Autodesk Fusion 360 part; units mm, degrees
ref_plane "WorkPlane3" through (0, 0, -38) normal (0, 0, 1) x (1, 0, 0)
sketch "Sketch6" plane through (0, 0, -38) normal (0, 0, 1) x (1, 0, 0)
  line L0 (-34.25, -21.25) -> (34.25, -21.25)
  line L1 (34.25, -21.25) -> (34.25, 21.25)
  line L2 (34.25, 21.25) -> (-34.25, 21.25)
  line L3 (-34.25, 21.25) -> (-34.25, -21.25)
extrude "Extrude6" add sketch "Sketch6" along normal blind 30
fillet "Fillet7" radius 2.5 4 edges at (-34.25, 21.25, -23) (34.25, 21.25, -23) (34.25, -21.25, -23) (-34.25, -21.25, -23)
ref_plane "WorkPlane4" through (0, 0, -8) normal (0, 0, 1) x (1, 0, 0)
sketch "Sketch7" plane through (0, 0, -8) normal (0, 0, 1) x (1, 0, 0)
  line L0 (-44.25, -31.25) -> (44.25, -31.25)
  line L1 (44.25, -31.25) -> (44.25, 90)
  line L2 (44.25, 90) -> (-44.25, 90)
  line L3 (-44.25, 90) -> (-44.25, -31.25)
extrude "Extrude7" add sketch "Sketch7" along normal blind 12
fillet "Fillet8" radius 7 4 edges at (-44.25, 90, -2) (44.25, 90, -2) (44.25, -31.25, -2) (-44.25, -31.25, -2)
sketch "Sketch8" plane through (0, 0, -8) normal (0, 0, 1) x (1, 0, 0)
  line L0 (-34.547, 90) -> (-11.5, 50.0814)
  arc A0 (-11.5, 50.0814) -> (11.5, 50.0814) centre (0, 70) ccw
  line L1 (11.5, 50.0814) -> (34.547, 90)
  line L2 (34.547, 90) -> (34.547, 95)
  line L3 (34.547, 95) -> (-34.547, 95)
  line L4 (-34.547, 95) -> (-34.547, 90)
extrude "Extrude8" cut sketch "Sketch8" along normal blind 12
fillet "Fillet9" radius 5 64 edges at (33.5178, -20.5178, -8) (0, -21.25, -8) (-33.5178, -20.5178, -8) (-34.25, 0, -8) (-33.5178, 20.5178, -8) (0, 21.25, -8) (33.5178, 20.5178, -8) (34.25, 0, -8) (34.25, 0, -8) (33.5178, 20.5178, -8) (0, 21.25, -8) (-33.5178, 20.5178, -8) (-34.25, 0, -8) (-33.5178, -20.5178, -8) (0, -21.25, -8) (33.5178, -20.5178, -8) (33.5178, 20.5178, -8) (34.25, 0, -8) (33.5178, -20.5178, -8) (0, -21.25, -8) (-33.5178, -20.5178, -8) (-34.25, 0, -8) (-33.5178, 20.5178, -8) (0, 21.25, -8) (0, 21.25, -8) (-33.5178, 20.5178, -8) (-34.25, 0, -8) (-33.5178, -20.5178, -8) (0, -21.25, -8) (33.5178, -20.5178, -8) (34.25, 0, -8) (33.5178, 20.5178, -8) (-33.5178, 20.5178, -8) (0, 21.25, -8) (33.5178, 20.5178, -8) (34.25, 0, -8) (33.5178, -20.5178, -8) (0, -21.25, -8) (-33.5178, -20.5178, -8) (-34.25, 0, -8) (-34.25, 0, -8) (-33.5178, -20.5178, -8) (0, -21.25, -8) (33.5178, -20.5178, -8) (34.25, 0, -8) (33.5178, 20.5178, -8) (0, 21.25, -8) (-33.5178, 20.5178, -8) (-33.5178, -20.5178, -8) (-34.25, 0, -8) (-33.5178, 20.5178, -8) (0, 21.25, -8) (33.5178, 20.5178, -8) (34.25, 0, -8) (33.5178, -20.5178, -8) (0, -21.25, -8) (0, -21.25, -8) (33.5178, -20.5178, -8) (34.25, 0, -8) (33.5178, 20.5178, -8) (0, 21.25, -8) (-33.5178, 20.5178, -8) (-34.25, 0, -8) (-33.5178, -20.5178, -8)
Could you check a few things on this model? Use its own coordinates, in mm. A direction names the side the tool comes from. Give positions to 0.01 mm unless a question says otherwise; leave off trailing zeros. Order: outer loops, then holes, each group sorted by start corner. A loop starts at its lowest first (then second) coordinate and runs counter-clockwise, first axis right, second up.
1. Suppose I cut it at B-B (y = 10). List the corners of the cut face in (x, z) for me, plus the area to 3 significant figures.
2. We'd pull the mould along X, two halves only. Please class faces 5 (the flat face through (-23, 70, -2)), 6 (the flat face through (0, 0, -38)), 7 (the cylindrical face through (-33.537, -20.498, -25.325)): pulls with the +X half, pulls with the -X half, needs draft (parallel to the pull), parting line crosses it, or undercut.
3. I need wall thicknesses on L1, parallel to X at y = 8, z = -22; L2, parallel to Z at x = -31.5, y = 62.5; L3, parallel to Y at x = 7, z = -32.5. Which ranges of each line are inside material? Lowest first, please.
4. For faces 1 (the flat face through (34.25, 0, -26)), 2 (the flat face through (23, 70, -2)), 3 (the flat face through (0, -21.25, -26)), 4 (the cylindrical face through (33.498, -20.537, -25.325)), which set-ups out of +Z, -Z, +X, -X, +Y, -Y let a thin tool reach every point of the face, with its end or its side?
5. Suppose I cut it at A-A (z = -15). List the corners of the cut face in (x, y) for me.
6. Suppose I cut it at D-D (z = -2). List the corners of the cut face in (x, y) for me.
7. Will these pins go through, and if not, where does the flat tip stop? P1, Ø1, axis at x = 33.5, y = 62.5, coming from the -Z side; P2, Ø5, axis at x = 32, z = -19, coming from the -Y side; P3, Ø20, axis at x = -5, z = -26, coming from the +Y side.
8. Suppose I cut it at C-C (x = -23). List the corners of the cut face in (y, z) for me.
Solved:
1. outline: (-44.25, -8) - (-39.25, -8) arc R5 cw to (-34.25, -13) - (-34.25, -38) - (34.25, -38) - (34.25, -13) arc R5 cw to (39.25, -8) - (44.25, -8) - (44.25, 4) - (-44.25, 4) - close
1. area: 3,130 mm2
2. face 5: undercut
2. face 6: needs draft
2. face 7: pulls with the -X half
3. L1: x = -34.25 to 34.25
3. L2: z = -8 to 4
3. L3: y = -21.25 to 21.25
4. face 1: -Z, +X, +Y, -Y
4. face 2: +Z, -Z, +Y
4. face 3: -Z, +X, -X, -Y
4. face 4: -Z, +X, -Y
5. outline: (-34.25, -18.75) arc R2.5 ccw to (-31.75, -21.25) - (31.75, -21.25) arc R2.5 ccw to (34.25, -18.75) - (34.25, 18.75) arc R2.5 ccw to (31.75, 21.25) - (-31.75, 21.25) arc R2.5 ccw to (-34.25, 18.75) - close
6. outline: (-44.25, -24.25) arc R7 ccw to (-37.25, -31.25) - (37.25, -31.25) arc R7 ccw to (44.25, -24.25) - (44.25, 83) arc R7 ccw to (37.25, 90) - (34.55, 90) - (11.5, 50.08) arc R23 cw to (-11.5, 50.08) - (-34.55, 90) - (-37.25, 90) arc R7 ccw to (-44.25, 83) - close
7. P1: stops at z = -8
7. P2: stops at y = -21.25
7. P3: stops at y = 21.25
8. outline: (-31.25, -8) - (-26.25, -8) arc R5 cw to (-21.25, -13) - (-21.25, -38) - (21.25, -38) - (21.25, -13) arc R5 cw to (26.25, -8) - (70, -8) - (70, 4) - (-31.25, 4) - close
